Geometry: see drawing. Coordinates: mm, zero at the bounding-box minimum. A direction names the side the tool comes from. Give positions to 0.01 mm unless a question says otherwise; leave off trailing zeros. Write each loop counter-clockwise with the first axis right and the second up, starting at its lowest first coordinate (ties: lowest second). Pieces come first, ordered by that corner, then holes. Notation, with made-up numbers: (29.25, -12) - (73.25, -12) arc R15 cw to (73.25, -2) - close; hole circle Ø2 at (-8.5, 6.5). An arc over 180 degrees is marked (long way). Use CSV: the item, a comma, the result in double quotes. Start each with the question number.
(1) Line query: probe 1 along Z at (x, y) = (208.5, 39.5); probe 2 along Y at (x, z) = (204.5, 147.5); probe 3 along X at (y, z) = (93.5, 88) (1 decimal). Output: solid intervals per line, ascending. Write a range as [from, to].
(2) Section A-A on x = 142.5. Output: boundary loops of the cut face in (y, z).
(3) First-contact query: pin 1 Ø1 at (x, z) = (229, 93) entering from +Y; pin 2 Ø1 at (x, z) = (89, 22.5) entering from +Y; pin 3 Ø8 at (y, z) = (71.5, 71) entering from +X. Flat tips, straight axial feed; report the tip coordinate or a pass-through.
(4) Reachability of the marked faces 1, 2, 3 and 4 from +Z, -Z, +X, -X, +Y, -Y: full face, straight path, thin tool, end or side. Return the list, or none.
(5) Section B-B on z = 143.5. Output: boundary loops of the cut face in (x, y) (1 decimal), and give its area (3 significant figures).
(6) Section D-D on z = 103.5. Output: boundary loops of the cut face in (x, y) (1 decimal), and give its area (3 significant figures).
(7) Section C-C on y = 87. Output: boundary loops of the cut face in (x, z), and give its area (3 significant figures).
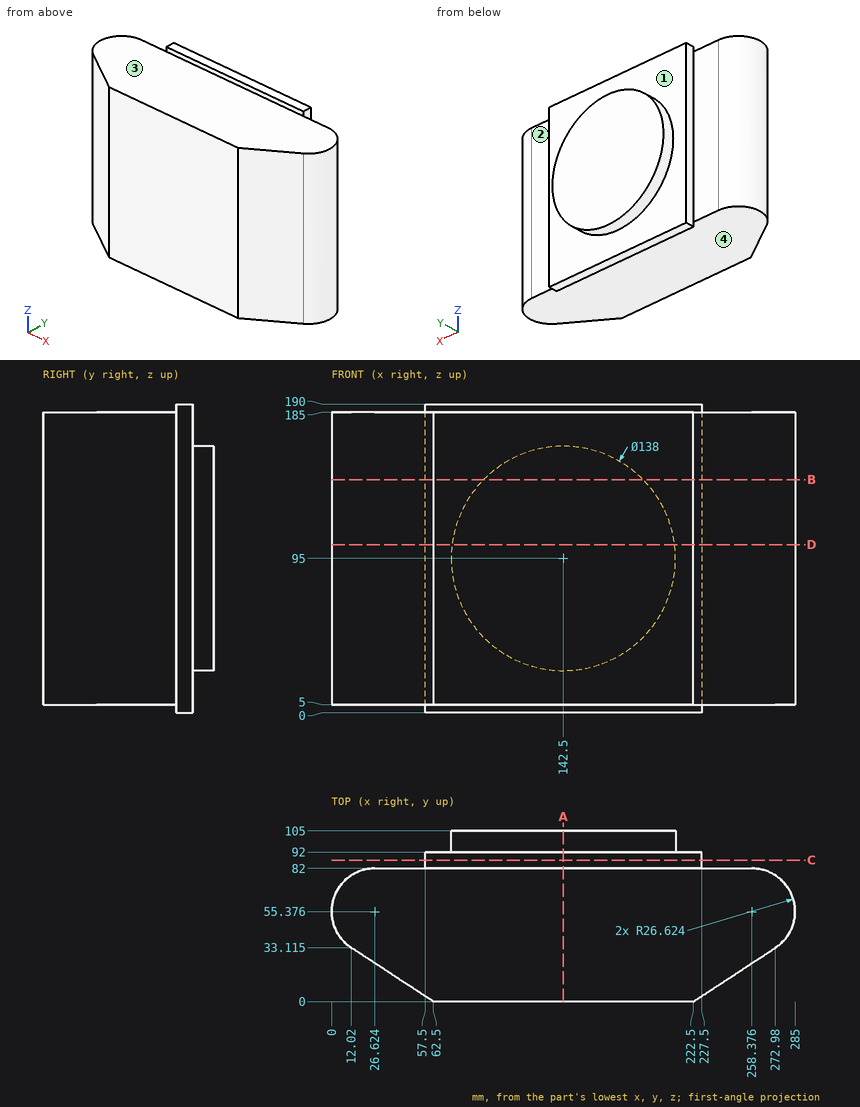
Check values:
1,probe 1,"z = [5, 185]"
1,probe 2,"y = [0, 92]"
1,probe 3,"x = [73.9, 211.1]"
2,outline,"(0, 5) - (82, 5) - (82, 0) - (92, 0) - (92, 26) - (105, 26) - (105, 164) - (92, 164) - (92, 190) - (82, 190) - (82, 185) - (0, 185) - close"
3,pin 1,"stops at y = 82"
3,pin 2,"stops at y = 92"
3,pin 3,"stops at x = 282.08"
4,face 1,"+Y"
4,face 2,"+Z, -Z, +X, +Y"
4,face 3,"+Z, +X, -X, -Y"
4,face 4,"-Z, +X, -X, -Y"
5,outline,"(12, 33.1) - (62.5, 0) - (222.5, 0) - (273, 33.1) arc R26.6 ccw to (258.4, 82) - (227.5, 82) - (227.5, 92) - (191.6, 92) - (191.6, 105) - (93.4, 105) - (93.4, 92) - (57.5, 92) - (57.5, 82) - (26.6, 82) arc R26.6 ccw to start"
5,area,"23,400 mm²"
6,outline,"(12, 33.1) - (62.5, 0) - (222.5, 0) - (273, 33.1) arc R26.6 ccw to (258.4, 82) - (227.5, 82) - (227.5, 92) - (211, 92) - (211, 105) - (74, 105) - (74, 92) - (57.5, 92) - (57.5, 82) - (26.6, 82) arc R26.6 ccw to start"
6,area,"23,900 mm²"
7,outline,"(57.5, 0) - (227.5, 0) - (227.5, 190) - (57.5, 190) - close"
7,area,"32,300 mm²"
